Check sheet for the drawn part. Datum: minimum x, y, z corner. Units: mm. A direction names the side the tool comes from. Coordinates: 2 decimals unless noted, no trailing zeros. Write each loop counter-clockwise with the first axis right and the second up, starting at its lowest first coordinate (ties: lowest second). Pieces come first, ordered by that corner, then holes. Notation, with made-up numbers: (42.5, 47) -> (77.5, 47) arc R28 cw to (77.5, 79) -> close; hole circle Ø2 at (67.25, 26.25). An arc over 180 degrees is marked (long way). Answer in a Markdown table with one row per item. Add a question column.
1. Mould release check, pull along Z, two halves, no side actions. Record for the marked faces 3, 4 and 5: pulls with the +Z half, pulls with the -Z half, needs draft (parallel to the pull), parting line crosses it, or undercut.
2. Scan lines: L1, parallel to Y at x = 18, z = 5; L2, parallel to Z at x = 25, y = 0.7; L3, parallel to X at y = 8.25, z = 25. Record each from-to range of solid material in increasing order. Write a range as from..to.
3. Depth check by flat-ended pin: P1, Ø1, axis at y = 8.5, z = 14.5, coming from the +X side; P2, Ø1.5, axis at x = 37, y = 4.5, coming from the +Z side; P3, Ø1, axis at x = 27, y = 13.5, coming from the -Z side. Enter the tip coordinate at first touch or a pass-through.
4. Set-up check for the marked faces 1 and 2: record each of +Z, -Z, +X, -X, +Y, -Y from which the full face is reachable in a straight line by a thin tool's end or side.
5. Cross-section at B-B on x = 25. Record the cut outline in (y, z), and give its area (3 significant figures).
6. Cross-section at C-C on x = 5. Record the cut outline in (y, z).
7. Cross-section at A-A on z = 25. Record the cut outline in (x, y).
8. Cross-section at D-D on y = 7.75. Record the cut outline in (x, z), and give its area (3 significant figures).
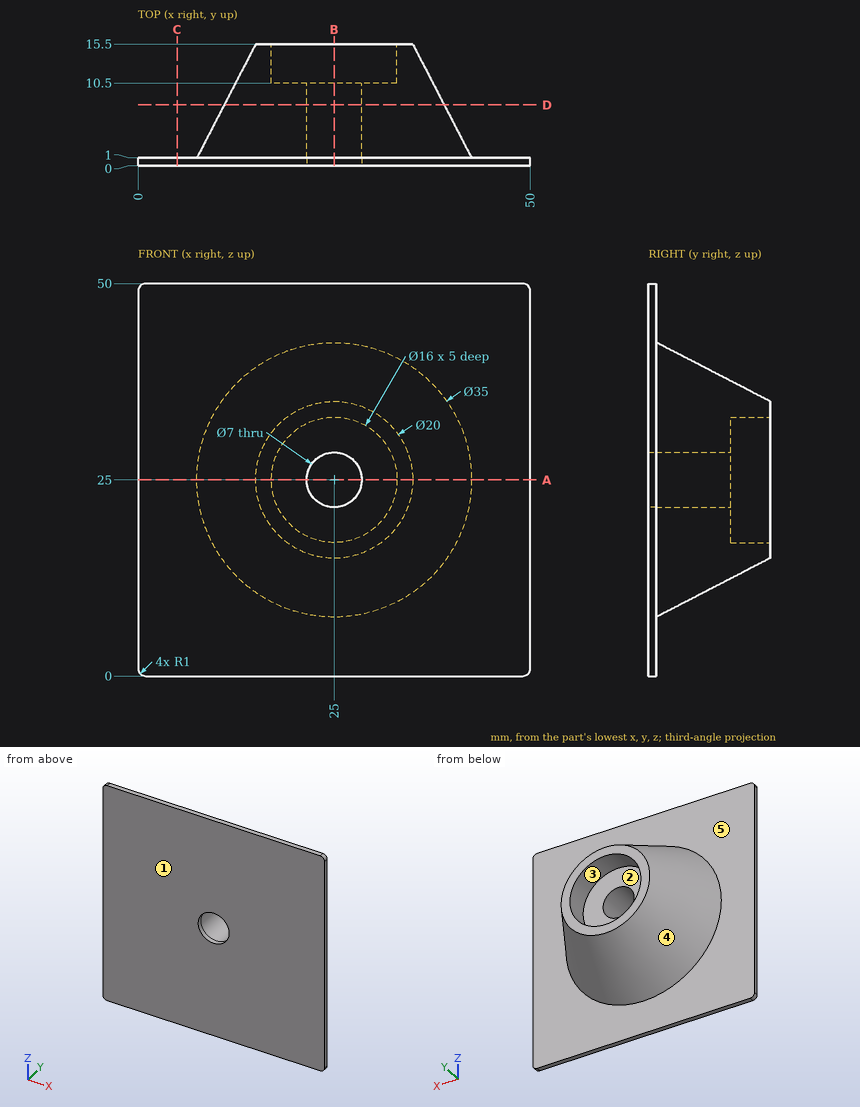
Results found:
| question | item | result |
|---|---|---|
| 1 | face 3 | undercut |
| 1 | face 4 | parting line crosses it |
| 1 | face 5 | needs draft |
| 2 | L1 | y = 0..1 |
| 2 | L2 | z = 0..21.5, 28.5..50 |
| 2 | L3 | x = 11.25..21.5, 28.5..38.75 |
| 3 | P1 | stops at x = 34.37 |
| 3 | P2 | stops at z = 36.12 |
| 3 | P3 | stops at z = 13.87 |
| 4 | face 1 | +Z, -Z, +X, -X, -Y |
| 4 | face 2 | +Y |
| 5 | outline | (0, 0) -> (1, 0) -> (1, 7.5) -> (15.5, 15) -> (15.5, 17) -> (10.5, 17) -> (10.5, 21.5) -> (0, 21.5) -> close; (0, 28.5) -> (10.5, 28.5) -> (10.5, 33) -> (15.5, 33) -> (15.5, 35) -> (1, 42.5) -> (1, 50) -> (0, 50) -> close |
| 5 | area | 295 mm^2 |
| 6 | outline | (0, 0) -> (1, 0) -> (1, 50) -> (0, 50) -> close |
| 7 | outline | (0, 0) -> (21.5, 0) -> (21.5, 10.5) -> (17, 10.5) -> (17, 15.5) -> (15, 15.5) -> (7.5, 1) -> (0, 1) -> close; (28.5, 0) -> (50, 0) -> (50, 1) -> (42.5, 1) -> (35, 15.5) -> (33, 15.5) -> (33, 10.5) -> (28.5, 10.5) -> close |
| 8 | outline | circle Ø28.02 at (25, 25); hole circle Ø7 at (25, 25) |
| 8 | area | 578 mm^2 |
